```python
from build123d import *

# Parameters (mm, degrees)
F0_W     = 103.5625115037
F0_H     = 94.215720892
F1_DEPTH = 25.4
F2_T     = -2
F4_DEPTH = 25.4


with BuildPart() as f1:
    # F0 (on Front) → F1 (new body)
    with BuildSketch(Plane.XZ):
        Rectangle(F0_W, F0_H)
    extrude(amount=F1_DEPTH)

    # F2
    f2_openings = [f1.faces().sort_by_distance(p)[0] for p in [
        (0, -25.4, 0),
    ]]
    offset(amount=F2_T, openings=f2_openings)

    # F3 (on face) → F4 (cut)
    with BuildSketch(Plane(origin=(0, 0, 0), x_dir=(-1, 0, 0), z_dir=(0, 1, 0))):
        with BuildLine():
            add(Edge.make_bspline(
                [(0, 15.3287509456), (2.8759838488, 19.61843277), (8.7431875053, 28.3696769384), (25.5477306115, 35.8525990524), (41.9020528727, 28.1543589695), (50.7457146307, 9.6766957358), (20.6699938695, -18.438481617), (0, -37.7610623837)],
                knots=[0, 0, 0, 0, 0.1637608356, 0.3340832995, 0.5015745629, 0.6574495816, 1, 1, 1, 1], degree=3))
            add(Edge.make_bspline(
                [(0, 15.3287509456), (-2.8759838488, 19.61843277), (-8.7431875053, 28.3696769384), (-25.5477306115, 35.8525990524), (-41.9020528727, 28.1543589695), (-50.7457146307, 9.6766957358), (-20.6699938695, -18.438481617), (0, -37.7610623837)],
                knots=[0, 0, 0, 0, 0.1637608356, 0.3340832995, 0.5015745629, 0.6574495816, 1, 1, 1, 1], degree=3))
        make_face()
    extrude(amount=-F4_DEPTH, mode=Mode.SUBTRACT)


solid = f1.part
```
Could you check a few things on this model? Use its own coordinates, in mm. A direction names the side the tool comes from. Round coordinates to 2 decimals unless told otherwise and drop trailing zeros. Loops run counter-clockwise (first coordinate to the right, second up) from the corner with the lowest first, then second, coordinate; pieces in that order, holes last. Notation, with made-up numbers: (35, -36) -> (49, -36) arc R14 cw to (49, -32) -> close; hole circle Ø1 at (61, 81.25). An arc over 180 degrees is marked (long way). One line per question, with ' | ' between items.
(1) If we section it at A-A on y = -9.5: List the corners of the cut face in (x, z) for me.
Model answer:
outline: (-51.78, -47.11) -> (51.78, -47.11) -> (51.78, 47.11) -> (-51.78, 47.11) -> close; hole (-49.78, -45.11) -> (49.78, -45.11) -> (49.78, 45.11) -> (-49.78, 45.11) -> close
(2) For faces 4 (the face through (-1, 0, 22)), 5 (the face through (-1, -2, 21)), which set-ups out of +Z, -Z, +X, -X, +Y, -Y let a thin tool reach every point of the face, with its end or its side?
Model answer:
face 4: +Z, -Z, +X, -X, +Y | face 5: -Y
(3) If we section it at B-B on z = 38: List the corners of the cut face in (x, y) for me.
Model answer:
outline: (-51.78, -25.4) -> (-49.78, -25.4) -> (-49.78, -2) -> (49.78, -2) -> (49.78, -25.4) -> (51.78, -25.4) -> (51.78, 0) -> (-51.78, 0) -> close
(4) Thinking about a two-plate mould opening in X: for faces 1 (the face through (-50, -25.4, 0)), 2 (the face through (-49.781, -14, -1)), 3 (the face through (51.781, -13, -1)), which applies, released by +X, released by -X, zero draft, split by the parting line, or undercut?
Model answer:
face 1: zero draft | face 2: undercut | face 3: released by +X
(5) For pin 1 Ø12 at (x, z) = (8, -25.5) entering from -Y, with a flat end and sliding along its axis, tell me the tip position at first contact or that it passes through.
Model answer:
pin 1: stops at y = -2
(6) If I drill on probe 1 along X at (y, z) = (-2.5, -34); probe 2 along Z at (x, y) = (20, -3.75); probe 3 along Y at (x, z) = (4, -42.5), over which ranges is the centre line in solid material (lowest first)?
Model answer:
probe 1: x = -51.78 to -49.78, 49.78 to 51.78 | probe 2: z = -47.11 to -45.11, 45.11 to 47.11 | probe 3: y = -2 to 0
